Here's how the part is built. I have some questions about the finished solid (model axes, mm). Round coordinates to 2 decimals unless told otherwise and drop trailing zeros. Write each loop counter-clockwise with the first axis right and the second up, starting at its lowest first coordinate (ties: lowest second). Pieces come first, ordered by that corner, then holes. Notation, with made-up numbers: (16, 57.25) -> (62, 57.25) arc R23 cw to (62, 74.25) -> close; hole circle Ø2 at (22, -18.75). An arc over 180 degrees is marked (long way). Answer in a Markdown table with one row per item.
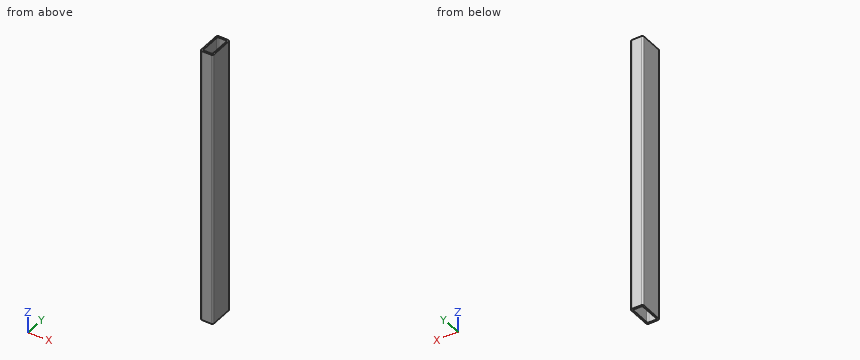
Autodesk Inventor part; units mm, degrees
ref_plane "YZ Plane" through (0, 0, 0) normal (1, 0, 0) x (0, 1, 0)
ref_plane "XZ Plane" through (0, 0, 0) normal (0, 1, 0) x (-1, 0, 0)
ref_plane "XY Plane" through (0, 0, 0) normal (0, 0, 1) x (1, 0, 0)
sketch "Sketch1" plane through (0, 0, 0) normal (0, 0, 1) x (1, 0, 0)
  line L0 (3.175, 0) -> (22.225, 0)
  line L1 (25.4, 3.175) -> (25.4, 47.625)
  line L2 (22.225, 50.8) -> (3.175, 50.8)
  line L3 (0, 47.625) -> (0, 3.175)
  arc A0 (3.175, 50.8) -> (0, 47.625) centre (3.175, 47.625) ccw
  arc A1 (25.4, 47.625) -> (22.225, 50.8) centre (22.225, 47.625) ccw
  arc A2 (22.225, 0) -> (25.4, 3.175) centre (22.225, 3.175) ccw
  arc A3 (0, 3.175) -> (3.175, 0) centre (3.175, 3.175) ccw
  line L4 (6.35, 47.625) -> (19.05, 47.625)
  line L5 (22.225, 44.45) -> (22.225, 6.35)
  line L6 (19.05, 3.175) -> (6.35, 3.175)
  line L7 (3.175, 6.35) -> (3.175, 44.45)
  arc A4 (6.35, 47.625) -> (3.175, 44.45) centre (6.35, 44.45) ccw
  arc A5 (22.225, 44.45) -> (19.05, 47.625) centre (19.05, 44.45) ccw
  arc A6 (3.175, 6.35) -> (6.35, 3.175) centre (6.35, 6.35) ccw
  arc A7 (19.05, 3.175) -> (22.225, 6.35) centre (19.05, 6.35) ccw
  point P0 (0, 0)
  point P1 (25.4, 0)
  point P2 (0, 50.8)
  dimension "d0" = 50.8
  dimension "d1" = 25.4
  dimension "d2" = 3.175
  dimension "d3" = 3.175
  dimension "d4" = 3.175
  dimension "d5" = 3.175
  dimension "d6" = 3.175
  dimension "d7" = 3.175
  dimension "d8" = 3.175
  dimension "d9" = 3.175
  dimension "d10" = 3.175
extrude "Extrusion1" add sketch "Sketch1" along normal blind 558.8
properties part number "O channel 22 inch"
1) For pin 1 (11.5 mm diameter, centred on y = 21.5, z = 187.5, fed in from -X); pin 2 (10 mm diameter, centred on x = 17, y = 38, fed in from -Z), each with a flat end and sliding along its axis, tell me the tip position at first contact or that it passes through.
Response:
| item | result |
|---|---|
| pin 1 | stops at x = 0 |
| pin 2 | passes through |
2) I want a section at B-B, the plane z = 184.5. List the corners of the cut face in (x, y) for me (3 decimals).
Response:
| item | result |
|---|---|
| outline | (0, 3.175) arc R3.175 ccw to (3.175, 0) -> (22.225, 0) arc R3.175 ccw to (25.4, 3.175) -> (25.4, 47.625) arc R3.175 ccw to (22.225, 50.8) -> (3.175, 50.8) arc R3.175 ccw to (0, 47.625) -> close; hole (3.175, 6.35) arc R3.175 ccw to (6.35, 3.175) -> (19.05, 3.175) arc R3.175 ccw to (22.225, 6.35) -> (22.225, 44.45) arc R3.175 ccw to (19.05, 47.625) -> (6.35, 47.625) arc R3.175 ccw to (3.175, 44.45) -> close |
3) I want a section at C-C, the plane y = 11. List the corners of the cut face in (x, z) for me (3 decimals).
Response:
| item | result |
|---|---|
| outline | (0, 0) -> (3.175, 0) -> (3.175, 558.8) -> (0, 558.8) -> close; (22.225, 0) -> (25.4, 0) -> (25.4, 558.8) -> (22.225, 558.8) -> close |
4) I need wall thicknesses on line 1 (X direction, y = 43.5, z = 107.5) (3 decimals); line 2 (Y direction, x = 14.75, z = 173) (3 decimals); line 3 (Y direction, x = 3.5, z = 314). Which ranges of each line are inside material? Lowest first, please. Write a range as [from, to].
Response:
| item | result |
|---|---|
| line 1 | x = [0, 3.175], [22.225, 25.4] |
| line 2 | y = [0, 3.175], [47.625, 50.8] |
| line 3 | y = [0, 4.95], [45.85, 50.8] |
5) I want a section at A-A, the plane x = 14.25. List the corners of the cut face in (y, z) for me (3 decimals), and give its area (3 significant figures).
Response:
| item | result |
|---|---|
| outline | (0, 0) -> (3.175, 0) -> (3.175, 558.8) -> (0, 558.8) -> close; (47.625, 0) -> (50.8, 0) -> (50.8, 558.8) -> (47.625, 558.8) -> close |
| area | 3,550 mm^2 |
